Could you check a few things on this drawing? It's one solid part, dimensions in mm from its lowest x, y, z. Give positions to 0.01 mm unless a question says otherwise; leave off trailing zeros. Loops run counter-clockwise (first coordinate to the right, second up) from the corner with the lowest first, then second, coordinate; pieces in that order, holes last. Notation, with made-up numbers: (35, 16) -> (40, 16) arc R18 ccw to (40, 46) -> close; hole circle Ø2 at (72, 12.25). An arc over 180 degrees is marked (long way). One line per question, with ' | ' between items.
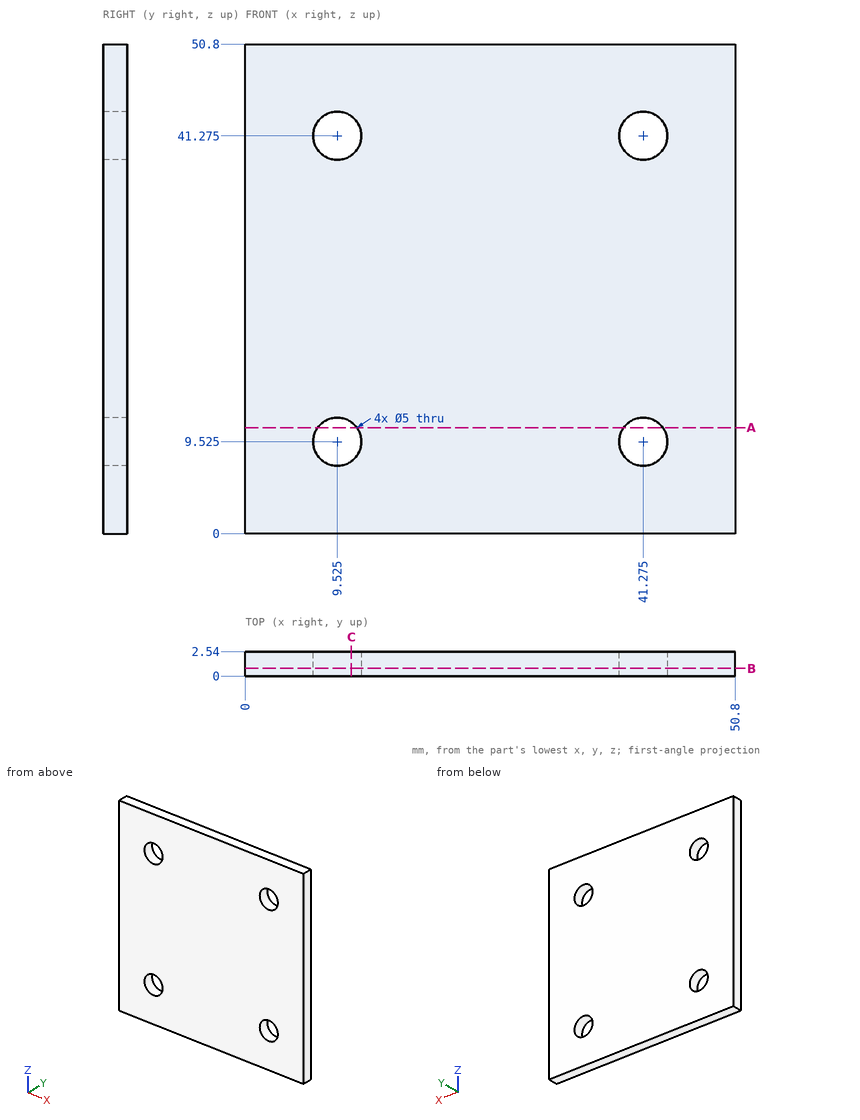
Q1. If we section it at B-B (y = 0.8): Write out the boundary of the cut face in (x, z) (3 decimals), plus the area to 3 significant figures.
Entries:
outline: (0, 0) -> (50.8, 0) -> (50.8, 50.8) -> (0, 50.8) -> close; hole circle Ø5 at (9.525, 9.525); hole circle Ø5 at (9.525, 41.275); hole circle Ø5 at (41.275, 9.525); hole circle Ø5 at (41.275, 41.275) | area: 2,500 mm²
Q2. If we section it at A-A (z = 11): Write out the boundary of the cut face in (x, y).
Entries:
outline: (0, 0) -> (7.51, 0) -> (7.51, 2.54) -> (0, 2.54) -> close; (11.54, 0) -> (39.26, 0) -> (39.26, 2.54) -> (11.54, 2.54) -> close; (43.29, 0) -> (50.8, 0) -> (50.8, 2.54) -> (43.29, 2.54) -> close
Q3. If we section it at C-C (x = 11): Write out the boundary of the cut face in (y, z).
Entries:
outline: (0, 0) -> (2.54, 0) -> (2.54, 7.51) -> (0, 7.51) -> close; (0, 11.54) -> (2.54, 11.54) -> (2.54, 39.26) -> (0, 39.26) -> close; (0, 43.29) -> (2.54, 43.29) -> (2.54, 50.8) -> (0, 50.8) -> close
Q4. For pin 1 Ø4.5 at (x, z) = (41.275, 9.525) entering from -Y, with a flat end and sliding along its axis, tell me the tip position at first contact or that it passes through.
Entries:
pin 1: through
Q5. If I drill on probe 1 along X at (y, z) = (2.05, 8); probe 2 along Z at (x, y) = (40, 0.85); probe 3 along Z at (x, y) = (40.5, 0.9), over which ranges is the centre line in solid material (lowest first)? Write a range as from..to.
Entries:
probe 1: 0..7.54, 11.51..39.29, 43.26..50.8 | probe 2: 0..7.37, 11.68..39.12, 43.43..50.8 | probe 3: 0..7.15, 11.9..38.9, 43.65..50.8
